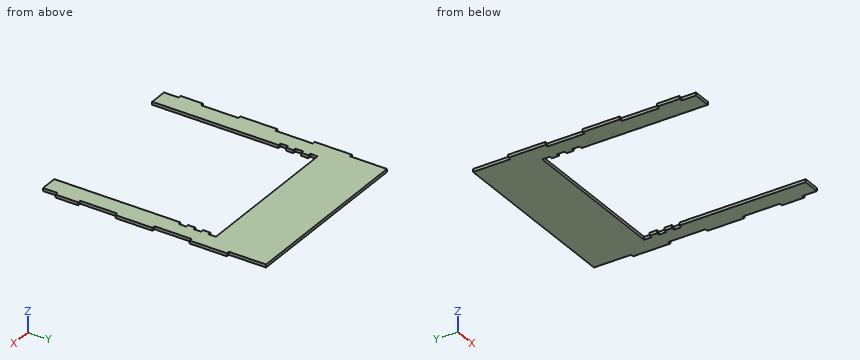
from build123d import *

# Parameters (mm, degrees)
F1_DEPTH = 4


with BuildPart() as f1:
    # F0 (on Top) → F1 (new body)
    with BuildSketch(Plane.XY):
        Polygon((-27, 0), (-4, 0), (-4, 19.556), (0, 19.556), (0, 50), (-4, 50), (-4, 100), (0, 100), (0, 150), (-4, 150), (-4, 200), (0, 200), (0, 250), (-4, 250), (-4, 300), (-251, 300), (-251, 250), (-255, 250), (-255, 200), (-251, 200), (-251, 150), (-255, 150), (-255, 100), (-251, 100), (-251, 50), (-255, 50), (-255, 19.556), (-251, 19.556), (-251, 0), (-227, 0), (-227, 170), (-231, 170), (-231, 180), (-227, 180), (-227, 190), (-231, 190), (-231, 200), (-227, 200), (-227, 210), (-231, 210), (-231, 220), (-227, 220), (-27, 220), (-23, 220), (-23, 210), (-27, 210), (-27, 200), (-23, 200), (-23, 190), (-27, 190), (-27, 180), (-23, 180), (-23, 170), (-27, 170), align=None)
    extrude(amount=F1_DEPTH)


solid = f1.part
Geometry check sheet. Reference: the model listing, model coordinates, mm. Round coordinates to 2 decimals unless told otherwise and drop trailing zeros. Order: outer loops, then holes, each group sorted by start corner. A loop starts at its lowest first (then second) coordinate and runs counter-clockwise, first axis right, second up. Notation, with made-up numbers: M 52,33 L 99,33 A12 cw 99,51 Z; hole C 71,-8 d8. An arc over 180 degrees is marked long. Answer in a Markdown table with one row per item. Add a question column.
Item 1: Depth check by flat-ended pin: pin 1 Ø1.5 at (x, z) = (-205.5, 1) entering from -Y; pin 2 Ø2 at (y, z) = (285, 1.5) entering from +X; pin 3 Ø1.2 at (x, z) = (-2.5, 2.5) entering from -Y. Enter the tip coordinate at first touch or a pass-through.
Item 2: Material ranges on L1, parallel to Y at x = -24.5, z = 2.9; L2, parallel to X at y = 17.5, z = 0.35; L3, parallel to X at y = 137, z = 3.6, recorded low to high. Write a range as [from, to].
Item 3: Sectioned sample at A-A, the plane y = 82. Enter the section's corners in (x, z), plus the area to 3 significant figures.
Item 4: Sectioned sample at B-B, the plane x = -52. Enter the section's corners in (y, z).
Filled in:
| question | item | result |
|---|---|---|
| 1 | pin 1 | stops at y = 220 |
| 1 | pin 2 | stops at x = -4 |
| 1 | pin 3 | stops at y = 19.56 |
| 2 | L1 | y = [0, 170], [180, 190], [200, 210], [220, 300] |
| 2 | L2 | x = [-251, -227], [-27, -4] |
| 2 | L3 | x = [-255, -227], [-27, 0] |
| 3 | outline | M -251,0 L -227,0 L -227,4 L -251,4 Z; M -27,0 L -4,0 L -4,4 L -27,4 Z |
| 3 | area | 188 mm² |
| 4 | outline | M 220,0 L 300,0 L 300,4 L 220,4 Z |
